```python
from build123d import *

# Parameters (mm, degrees)
F1_DEPTH = 20
F2_SIZE  = 5
F3_R     = 5
F4_R     = 10
F4_W     = 6
F4_H     = 6
F5_DEPTH = 54.4


with BuildPart() as f1:
    # F0 (on Top) → F1 (new body)
    with BuildSketch(Plane.XY):
        Polygon((-22.5, -22.5), (22.5, -22.5), (22.5, 22.5), (-22.5, 22.5), (-22.5, 10), (-42.5, 10), (-42.5, -10), (-22.5, -10), align=None)
    extrude(amount=F1_DEPTH)

    # F2
    f2_edges = [f1.edges().sort_by_distance(p)[0] for p in [
        (-22.5, -22.5, 10),
        (-22.5, 22.5, 10),
    ]]
    chamfer(f2_edges, length=F2_SIZE)

    # F3
    f3_edges = [f1.edges().sort_by_distance(p)[0] for p in [
        (22.5, 0, 20),
    ]]
    fillet(f3_edges, radius=F3_R)

    # F4 (on face) → F5 (cut, symmetric)
    with BuildSketch(Plane.XZ.offset(10)):
        with Locations((-0.5, 20)):
            Circle(F4_R)
        with Locations((-32.5, 10)):
            Rectangle(F4_W, F4_H)
    extrude(amount=F5_DEPTH, both=True, mode=Mode.SUBTRACT)


solid = f1.part
```
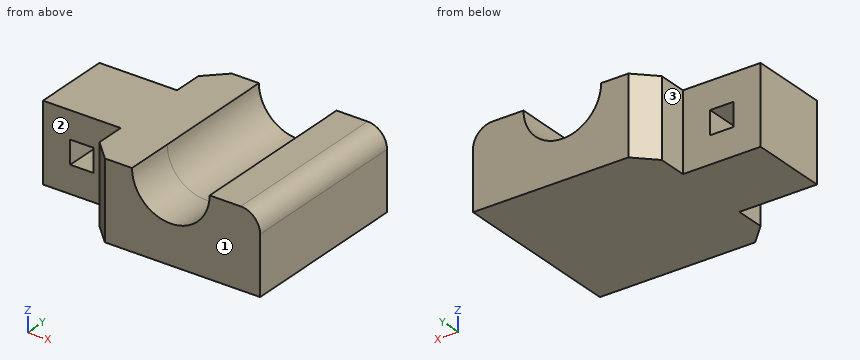
Model file for the job. Use its own axes, mm. Face numbers are marked on the shaded views. A direction names the side the tool comes from. Coordinates: 2 decimals unless noted, no trailing zeros. Write each loop counter-clockwise with the first axis right and the second up, starting at its lowest first coordinate (ties: lowest second). Pieces come first, ordered by that corner, then holes. Notation, with made-up numbers: (81.5, 77) - (111.5, 77) arc R15 cw to (111.5, 90) - close; hole circle Ø3 at (66, 77). An arc over 180 degrees is marked (long way). One line per question, with ' | ' between items. Start each with the question number.
Q1. Cut at B-B, the plane z = 2.5. List the corners of the cut face in (x, y).
Q2. Drill centre lines: line 1 (X direction, y = 21.5, z = 16.75); line 2 (X direction, y = -3, z = 17.5); line 3 (Z direction, x = -0.5, y = -2.5). Where is each one in solid material? Low to high. Write a range as [from, to].
Q3. Pin check, flat tips, straight feed: pin 1 (8 mm diameter, centred on y = 12, z = 5, fed in from -X); pin 2 (1 mm diameter, centred on x = -19, z = 3.5, fed in from +Y); pin 3 (10 mm diameter, centred on x = -37, z = 6.5, fed in from +Y); pin 4 (4 mm diameter, centred on y = -12.5, z = 10, fed in from -X). Stop position of each tip, or through.
Q4. Cut at C-C, the plane y = 16. List the corners of the cut face in (x, z).
Q5. Cut at D-D, the plane x = -0.5. List the corners of the cut face in (y, z).
Q6. 3-axis set-ups, long thin cutter, end or side, ignore diameter. For the marked faces 1, 2 and 3: which of +Z, -Z, +X, -X, +Y, -Y reach the whole face in a straight line?
Q7. Cut at A-A, the plane y = 7. List the corners of the cut face in (x, z).
Answer below:
1) outline: (-42.5, -10) - (-22.5, -10) - (-22.5, -17.5) - (-17.5, -22.5) - (22.5, -22.5) - (22.5, 22.5) - (-17.5, 22.5) - (-22.5, 17.5) - (-22.5, 10) - (-42.5, 10) - close
2) line 1: [-18.5, -9.96], [8.96, 22.18] | line 2: [-42.5, -10.18], [9.18, 21.83] | line 3: [0, 10]
3) pin 1: x = -42.5 | pin 2: y = 21.5 | pin 3: y = 10 | pin 4: x = -22.5
4) outline: (-22.5, 0) - (22.5, 0) - (22.5, 15) arc R5 ccw to (17.5, 20) - (9.5, 20) arc R10 cw to (-10.5, 20) - (-22.5, 20) - close
5) outline: (-22.5, 0) - (22.5, 0) - (22.5, 10) - (-22.5, 10) - close
6) face 1: +Z, -Z, +X, -X, -Y | face 2: +Z, -Z, -X, -Y | face 3: +Z, -Z, -X, +Y
7) outline: (-42.5, 0) - (22.5, 0) - (22.5, 15) arc R5 ccw to (17.5, 20) - (9.5, 20) arc R10 cw to (-10.5, 20) - (-42.5, 20) - close; hole (-35.5, 7) - (-29.5, 7) - (-29.5, 13) - (-35.5, 13) - close
